from build123d import *

# Parameters (mm, degrees)
F0_R     = 19.1968698124
F0_R_2   = 9.3617301333
F1_DEPTH = 38.1
F2_R     = 7.6435509614
F3_DEPTH = 38.1
F4_W     = 45.4035978764
F4_H     = 66.3013830781
F5_DEPTH = 114.3


with BuildPart() as f1:
    # F0 (on Front) → F1 (new body, symmetric)
    with BuildSketch(Plane.XZ):
        Circle(F0_R)
        Circle(F0_R_2, mode=Mode.SUBTRACT)
    extrude(amount=F1_DEPTH, both=True)

    # F2 (on Front) → F3 (join, symmetric)
    with BuildSketch(Plane.XZ):
        with BuildLine():
            Line((-20.3485637903, 45.8143912256), (-20.3485637903, 0))
            Line((-20.3485637903, 0), (20.3485637903, 0))
            Line((20.3485637903, 0), (20.3485637903, 45.8143912256))
            Line((20.3485637903, 45.8143912256), (19.6841994122, 45.8143912256))
            ThreePointArc((19.6841994122, 45.8143912256), (0, 65.4985906377), (-19.6841994122, 45.8143912256))
            Line((-19.6841994122, 45.8143912256), (-20.3485637903, 45.8143912256))
        make_face()
        with Locations((0, 45.8143912256)):
            Circle(F2_R, mode=Mode.SUBTRACT)
    extrude(amount=F3_DEPTH, both=True)

    # F4 (on Right) → F5 (cut, symmetric)
    with BuildSketch(Plane.YZ):
        with Locations((1.2458292767, 33.150691539)):
            Rectangle(F4_W, F4_H)
    extrude(amount=F5_DEPTH, both=True, mode=Mode.SUBTRACT)


solid = f1.part
CAD build for the part. Positions are in the model's coordinates, mm. A direction names the side the tool comes from. Round coordinates to 2 decimals unless told otherwise and drop trailing zeros. Loops run counter-clockwise (first coordinate to the right, second up) from the corner with the lowest first, then second, coordinate; pieces in that order, holes last.
(1) Which spindle directions (+Z, -Z, +X, -X, +Y, -Y) get a long thin tool onto all of the face, cutting with end or side? Do faces 1 (the flat face through (0, -30, 0)), 2 (the flat face through (-20.349, 31, 23)), 3 (the flat face through (0, -21.456, 32)). Say none if no direction does.
(2) Cut at D-D (y = -13.5). Give the cut face in (x, z).
(3) Two-plate mould, pull along X, no slides. Class faces 4 (the flat face through (20.349, -30, 23)), 5 (the flat face through (-20.349, -30, 23)), 6 (the flat face through (0, 31, 0)): +X half, -X half, draft (parallel to the pull), parting line (faces both ways), or undercut.
(4) Cut at A-A (x = 0). Give the cut face in (y, z), plus the area to 3 significant figures.
(5) Wall check: line 1 along Z through (x, y) = (0, -32.5); line 2 along Y through (x, z) = (6, 2.5); line 3 along Z through (x, y) = (-1, 31). Give the ranges that are in metal, low to high.
(6) Cut at C-C (x = 11). Give the cut face in (y, z).
(7) Drop flat-ended pins along their axis: pin 1 (14 mm diameter, centred on x = 0, z = 45.81, fed in from +Y); pin 2 (3 mm diameter, centred on x = 13, y = -1, fed in from +Z); pin 3 (4 mm diameter, centred on x = -10.5, y = -23.5, fed in from -Z); pin 4 (8 mm diameter, centred on y = 21, z = 33, fed in from -X). Give the stop position or say it passes through.
(8) Cut at B-B (y = -32). Give the cut face in (x, z), plus the area to 3 significant figures.
Findings below:
1. face 1: +Y, -Y
1. face 2: +Z, -Z, -X, +Y, -Y
1. face 3: +Z, +X, -X
2. outline: (-19.2, 0) arc R19.2 ccw to (19.2, 0) - (9.36, 0) arc R9.36 cw to (-9.36, 0) - close
3. face 4: +X half
3. face 5: -X half
3. face 6: undercut
4. outline: (-38.1, -19.2) - (38.1, -19.2) - (38.1, -9.36) - (-38.1, -9.36) - close; (-38.1, 0) - (-21.46, 0) - (-21.46, 38.17) - (-38.1, 38.17) - close; (-38.1, 53.46) - (-21.46, 53.46) - (-21.46, 65.5) - (-38.1, 65.5) - close; (23.95, 0) - (38.1, 0) - (38.1, 38.17) - (23.95, 38.17) - close; (23.95, 53.46) - (38.1, 53.46) - (38.1, 65.5) - (23.95, 65.5) - close
4. area: 2,300 mm2
5. line 1: z = -19.2 to -9.36, 0 to 38.17, 53.46 to 65.5
5. line 2: y = -38.1 to -21.46, 23.95 to 38.1
5. line 3: z = -19.17 to -9.31, 0 to 38.24, 53.39 to 65.47
6. outline: (-38.1, -15.73) - (38.1, -15.73) - (38.1, 62.14) - (23.95, 62.14) - (23.95, 0) - (-21.46, 0) - (-21.46, 62.14) - (-38.1, 62.14) - close
7. pin 1: passes through
7. pin 2: stops at z = 0
7. pin 3: stops at z = -17.21
7. pin 4: stops at x = -20.35
8. outline: (-20.35, 0) - (-19.2, 0) arc R19.2 ccw to (19.2, 0) - (20.35, 0) - (20.35, 45.81) - (19.68, 45.81) arc R19.68 ccw to (-19.68, 45.81) - (-20.35, 45.81) - close; hole (-9.36, 0) arc R9.36 ccw to (9.36, 0) - close; hole circle Ø15.29 at (0, 45.81)
8. area: 2,730 mm2
